Autodesk Inventor part; units mm, degrees
ref_plane "YZ Plane" through (0, 0, 0) normal (1, 0, 0) x (0, 1, 0)
ref_plane "XZ Plane" through (0, 0, 0) normal (0, 1, 0) x (-1, 0, 0)
ref_plane "XY Plane" through (0, 0, 0) normal (0, 0, 1) x (1, 0, 0)
sketch "Sketch1" plane through (0, 0, 0) normal (0, 0, 1) x (1, 0, 0)
  line L0 (-46.75, 20.4) -> (46.75, 20.4)
  line L1 (46.75, 20.4) -> (46.75, -20.4)
  line L2 (46.75, -20.4) -> (-46.75, -20.4)
  line L3 (-46.75, -20.4) -> (-46.75, 20.4)
  line L4 (-31.65, 16) -> (-24.85, 16) construction
  line L5 (-31.65, 14.4) -> (-24.85, 14.4)
  line L6 (-24.85, 17.6) -> (-31.65, 17.6)
  arc A0 (-31.65, 17.6) -> (-31.65, 14.4) centre (-31.65, 16) ccw
  arc A1 (-24.85, 14.4) -> (-24.85, 17.6) centre (-24.85, 16) ccw
  line L7 (-31.65, -16) -> (-24.85, -16) construction
  line L8 (-31.65, -17.6) -> (-24.85, -17.6)
  line L9 (-24.85, -14.4) -> (-31.65, -14.4)
  arc A2 (-31.65, -14.4) -> (-31.65, -17.6) centre (-31.65, -16) ccw
  arc A3 (-24.85, -17.6) -> (-24.85, -14.4) centre (-24.85, -16) ccw
  line L10 (35.35, 16) -> (42.15, 16) construction
  line L11 (35.35, 14.4) -> (42.15, 14.4)
  line L12 (42.15, 17.6) -> (35.35, 17.6)
  arc A4 (35.35, 17.6) -> (35.35, 14.4) centre (35.35, 16) ccw
  arc A5 (42.15, 14.4) -> (42.15, 17.6) centre (42.15, 16) ccw
  line L13 (35.35, -16) -> (42.15, -16) construction
  line L14 (35.35, -17.6) -> (42.15, -17.6)
  line L15 (42.15, -14.4) -> (35.35, -14.4)
  arc A6 (35.35, -14.4) -> (35.35, -17.6) centre (35.35, -16) ccw
  arc A7 (42.15, -17.6) -> (42.15, -14.4) centre (42.15, -16) ccw
  line L16 (-28.25, 16) -> (-28.25, -16) construction
  line L17 (-28.25, -16) -> (38.75, -16) construction
  circle A8 centre (28.7, 0) radius 1.6
  circle A9 centre (-28.3, 0) radius 1.6
  circle A10 centre (38.15, 0) radius 0.6
  circle A11 centre (19.15, 0) radius 0.6
  circle A12 centre (0.15, 0) radius 0.6
  circle A13 centre (-18.85, 0) radius 0.6
  circle A14 centre (-37.85, 0) radius 0.6
  point P0 (0, 0)
  point P1 (0, 20.4)
  point P2 (-46.75, 0)
  point P3 (38.75, 16)
  point P4 (-28.25, 0)
  dimension "d0" = 40.8
  dimension "d1" = 93.5
  dimension "d2" = 3.2
  dimension "d3" = 3.2
  dimension "d4" = 3.2
  dimension "d5" = 3.2
  dimension "d6" = 32
  dimension "d7" = 67
  dimension "d8" = 4.6
  dimension "d9" = 6.8
  dimension "d10" = 3.2
  dimension "d11" = 57
  dimension "d13" = 1.2
  dimension "d14" = 8.6
  dimension "d15" = 1.2
  dimension "d16" = 1.2
  dimension "d17" = 1.2
  dimension "d18" = 1.2
  dimension "d20" = 19
  dimension "d21" = 19
  dimension "d22" = 19
  dimension "d23" = 19
  dimension "d27" = 18.05
extrude "PCB SiPM 4CH corta" add sketch "Sketch1" along normal mid plane 1.6
equation "\"d21\" = d20"
equation "\"d22\" = d20"
equation "\"d23\" = d20"
properties part number "PCB SiPM 4CH corta" material "Phenolic Resin"
Design review of the part built by this model. Coordinates are the model's own, in mm. A direction names the side the tool comes from. Coordinates: 2 decimals unless noted, no trailing zeros. Loops run counter-clockwise (first coordinate to the right, second up) from the corner with the lowest first, then second, coordinate; pieces in that order, holes last. Notation, with made-up numbers: M -26.75,-2.75 L 31.25,-2.75 A16 ccw 31.25,24.25 Z; hole C -27,75 d11. An arc over 180 degrees is marked long. Use one line per item in the form item = value.
(1) For line 1 along Y through (x, z) = (38.15, 0.55); line 2 along Y through (x, z) = (36, -0.4); line 3 along Y through (x, z) = (-37.85, 0.2), list the stretches that pass through material, from the lowest coordinate up. Write a range as from..to.
Return value:
line_1 = -20.4..-17.6, -14.4..-0.6, 0.6..14.4, 17.6..20.4
line_2 = -20.4..-17.6, -14.4..14.4, 17.6..20.4
line_3 = -20.4..-0.6, 0.6..20.4
(2) For faces 4 (the face through (-46.75, 0, 0)), 5 (the face through (-28, 14.4, 0)), list the 3-axis set-ups (+Z, -Z, +X, -X, +Y, -Y) from which the entire face can be reached by the end or side of a thin tool; tool diameter is ignored.
Return value:
face_4 = +Z, -Z, -X, +Y, -Y
face_5 = +Z, -Z
(3) Consider section B-B (z = 0.25). Give the number of separate pieces and of enclosed holes in the cut face, and give its area (3 significant figures).
Return value:
separate_pieces = 1
enclosed_holes = 11
area = 3,670 mm2
(4) Consider section C-C (y = 16). Write out the cut boundary in (x, z), and give its area (3 significant figures).
Return value:
outline = M -46.75,-0.8 L -33.25,-0.8 L -33.25,0.8 L -46.75,0.8 Z; M -23.25,-0.8 L 33.75,-0.8 L 33.75,0.8 L -23.25,0.8 Z; M 43.75,-0.8 L 46.75,-0.8 L 46.75,0.8 L 43.75,0.8 Z
area = 118 mm2
(5) Draft analysis for pull direction Y (two halves, no side actions). For faces 1 (the face through (1, -20.4, 0)), 2 (the face through (-33.25, 15.96, -0.01)), 3 (the face through (-1, 0, -0.8)), state which applies: pulls with the +Y half, pulls with the -Y half, needs draft (parallel to the pull), parting line crosses it, or undercut.
Return value:
face_1 = pulls with the -Y half
face_2 = undercut
face_3 = needs draft
(6) Consider section A-A (x = -28.3). Write out the cut boundary in (y, z), and give its area (3 significant figures).
Return value:
outline = M -20.4,-0.8 L -17.6,-0.8 L -17.6,0.8 L -20.4,0.8 Z; M -14.4,-0.8 L -1.6,-0.8 L -1.6,0.8 L -14.4,0.8 Z; M 1.6,-0.8 L 14.4,-0.8 L 14.4,0.8 L 1.6,0.8 Z; M 17.6,-0.8 L 20.4,-0.8 L 20.4,0.8 L 17.6,0.8 Z
area = 49.9 mm2
